Read the model definition and answer for the solid it produces. Units are mm, in the model's axes. A direction names the side the tool comes from. Round coordinates to 2 decimals unless told otherwise and drop trailing zeros. Order: outer loops, then holes, each group sorted by start corner. A loop starts at its lowest first (then second) coordinate and runs counter-clockwise, first axis right, second up. Notation, with made-up numbers: M 81.5,2 L 90.5,2 A23 cw 90.5,38 Z; hole C 23.25,21 d8. An arc over 180 degrees is marked long. Answer as CSV lines item,"result".
Autodesk Inventor part; units mm, degrees
ref_plane "YZ Plane" through (0, 0, 0) normal (1, 0, 0) x (0, 1, 0)
ref_plane "XZ Plane" through (0, 0, 0) normal (0, 1, 0) x (-1, 0, 0)
ref_plane "XY Plane" through (0, 0, 0) normal (0, 0, 1) x (1, 0, 0)
sketch "스케치1" plane through (0, 0, 0) normal (1, 0, 0) x (0, 1, 0)
  line L0 (0, 0) -> (51, 0)
  line L1 (51, 0) -> (51, -50)
  line L2 (51, -50) -> (0, -50)
  line L3 (0, -50) -> (0, 0)
  line L4 (0, -25) -> (30, -25)
  line L5 (0, -10) -> (14.5, -10)
  line L6 (0, -40) -> (14.5, -40)
  line L7 (14.5, -10) -> (45.5, -10)
  line L8 (14.5, -40) -> (45.5, -40)
  circle A0 centre (45.5, -10) radius 1.75
  circle A1 centre (14.5, -10) radius 1.75
  circle A2 centre (45.5, -40) radius 1.75
  circle A3 centre (14.5, -40) radius 1.75
  circle A4 centre (30, -25) radius 11.05
  line L9 (3, -50) -> (3, 0)
  dimension "d0" = 51
  dimension "d1" = 50
  dimension "d2" = 30
  dimension "d3" = 14.5
  dimension "d4" = 14.5
  dimension "d5" = 31
  dimension "d6" = 31
  dimension "d7" = 3.5
  dimension "d8" = 3.5
  dimension "d9" = 3.5
  dimension "d10" = 3.5
  dimension "d11" = 22.1
extrude "돌출1" add sketch "스케치1" along normal blind 3 contours L0 L1 L2 L9
extrude "돌출2" add sketch "스케치1" along normal blind 53 contours L0 L9 L5 L3 | L5 L9 L4 L3 | L4 L9 L6 L3 | L6 L9 L2 L3
sketch "스케치2" plane through (0, 0, -50) normal (0, -1, 0) x (1, 0, 0)
  line L0 (53, 0) -> (53, 10)
  line L1 (53, 0) -> (53, 50)
  line L2 (53, 10) -> (42, 10)
  line L3 (53, 50) -> (53, 40)
  line L4 (53, 40) -> (42, 40)
  arc A0 (12, 12.1) -> (12, 7.9) centre (12, 10) ccw
  arc A1 (42, 7.9) -> (42, 12.1) centre (42, 10) ccw
  arc A2 (12, 42.1) -> (12, 37.9) centre (12, 40) ccw
  arc A3 (42, 37.9) -> (42, 42.1) centre (42, 40) ccw
  line L5 (12, 12.1) -> (42, 12.1)
  line L6 (12, 37.9) -> (42, 37.9)
  line L7 (42, 42.1) -> (12, 42.1)
  line L8 (12, 7.9) -> (42, 7.9)
  point P0 (0, 50)
  dimension "d16" = 10
  dimension "d17" = 11
  dimension "d18" = 10
  dimension "d19" = 11
  dimension "d22" = 4.2
  dimension "d23" = 4.2
  dimension "d24" = 4.2
  dimension "d25" = 4.2
extrude "돌출3" cut sketch "스케치2" against normal blind 3
properties part number "모터 브라켓"
Item 1: A cutting plane is placed at C-C, the plane x = 28.5. Determine the outline of the cut face in (y, z), and give its area (3 significant figures).
Ans:
outline,"M 0,-50 L 3,-50 L 3,-42.1 L 0,-42.1 Z; M 0,-37.9 L 3,-37.9 L 3,-12.1 L 0,-12.1 Z; M 0,-7.9 L 3,-7.9 L 3,0 L 0,0 Z"
area,"125 mm2"
Item 2: Flat-ended cylindrical pins translate along their axes: pin 1 (1.5 mm diameter, centred on y = 39.5, z = -42.5, fed in from +X); pin 2 (4 mm diameter, centred on x = 19.5, z = -13.5, fed in from +Y). Find the tip coordinate at first contact, or state that the pin passes through.
Ans:
pin 1,"x = 3"
pin 2,"y = 3"
Item 3: A cutting plane is placed at D-D, the plane y = 14.5. Determine the outline of the cut face in (x, z), and give its area (3 significant figures).
Ans:
outline,"M 0,-50 L 3,-50 L 3,-41.75 L 0,-41.75 Z; M 0,-38.25 L 3,-38.25 L 3,-11.75 L 0,-11.75 Z; M 0,-8.25 L 3,-8.25 L 3,0 L 0,0 Z"
area,"129 mm2"
Item 4: A tool of negligible diameter and unlimited length cuts with its end or side. For faces 4 (the face through (44.1, 1.5, -40)), 5 (the face through (3, 16, -25)), 6 (the face through (1.5, 15.4, -11.5)), from which of +Z, -Z, +X, -X, +Y, -Y can it reach the whole face along a straight path? Write none if from no direction.
Ans:
face 4,"+Y, -Y"
face 5,"+Z, -Z, +X, +Y"
face 6,"+X, -X"
Item 5: Determine the mould class of faces 1 (the face through (28, 3, -25)), 2 (the face through (27, 1, -42.1)), 3 (the face through (1.48, 21.86, -32.47)) for opening direction Y: +Y half, -Y half, draft (parallel to the pull), parting line (faces both ways), or undercut.
Ans:
face 1,"+Y half"
face 2,"draft"
face 3,"undercut"
Item 6: Find the intervals of material crossed by probe 1 along Y at (x, z) = (1, -10); probe 2 along Z at (x, y) = (1.8, 45.5); probe 3 along Y at (x, z) = (33, -31), in increasing order. Write a range as [from, to].
Ans:
probe 1,"[0, 12.75], [16.25, 43.75], [47.25, 51]"
probe 2,"[-50, -41.75], [-38.25, -11.75], [-8.25, 0]"
probe 3,"[0, 3]"
Item 7: A cutting plane is placed at B-B, the plane z = -25. Determine the outline of the cut face in (x, y).
Ans:
outline,"M 0,0 L 53,0 L 53,3 L 3,3 L 3,18.95 L 0,18.95 Z; M 0,41.05 L 3,41.05 L 3,51 L 0,51 Z"
Item 8: A cutting plane is placed at A-A, the plane y = 30. Determine the outline of the cut face in (x, z).
Ans:
outline,"M 0,-50 L 3,-50 L 3,-36.05 L 0,-36.05 Z; M 0,-13.95 L 3,-13.95 L 3,0 L 0,0 Z"
